The model under review builds one solid part; all positions refer to its coordinate system, in mm. A direction names the side the tool comes from. Round coordinates to 2 decimals unless told otherwise and drop trailing zeros. Order: outer loops, then holes, each group sorted by start corner. A loop starts at its lowest first (then second) coordinate and runs counter-clockwise, first axis right, second up.
```python
from build123d import *

# Parameters (mm, degrees)
SKETCH_1_R           = 22
SKETCH_1_R_2         = 17
EXTRUDE_1_DEPTH      = 9
SKETCH_2_R           = 22
EXTRUDE_2_DEPTH      = 3
SKETCH_3_R           = 1
CUT_EXTRUDE_1_DEPTH  = 3
CUT_EXTRUDE_2_DEPTH  = 25
SKETCH_5_R           = 4
CUT_EXTRUDE_3_DEPTH  = 10
FILLET_1_R           = 10
FILLET_2_R           = 10
SKETCH_7_R           = 25
SKETCH_7_R_2         = 22
EXTRUDE_3_DEPTH      = 30
EXTRUDE_4_DEPTH      = 4
SKETCH_9_R           = 38.67245247
CUT_EXTRUDE_4_DEPTH  = 1
SKETCH_10_R          = 25
SKETCH_10_R_2        = 22
EXTRUDE_5_DEPTH      = 13.5
SKETCH_11_R          = 23
CUT_EXTRUDE_5_DEPTH  = 10.5
CHAMFER_2_SIZE       = 1
SKETCH_12_R          = 23
CUT_EXTRUDE_6_DEPTH  = 18
SKETCH_13_R          = 39.83087954
CUT_EXTRUDE_7_DEPTH  = 2.5
SKETCH_14_R          = 15
CUT_EXTRUDE_8_DEPTH  = 0.5
SKETCH_15_R          = 25
SKETCH_15_R_2        = 23
EXTRUDE_6_DEPTH      = 2
SKETCH_16_R          = 20
CUT_EXTRUDE_9_DEPTH  = 9
SKETCH_17_R          = 20
SKETCH_17_R_2        = 1
SKETCH_17_R_3        = 4
EXTRUDE_7_DEPTH      = 2.5
SKETCH_18_R          = 1.5
CUT_EXTRUDE_10_DEPTH = 21.5
CUT_EXTRUDE_11_DEPTH = 21.5


with BuildPart() as part:
    # 草图1 → 凸台-拉伸1 (new body)
    with BuildSketch(Plane.XY):
        Circle(SKETCH_1_R)
        Circle(SKETCH_1_R_2, mode=Mode.SUBTRACT)
    extrude(amount=EXTRUDE_1_DEPTH)

    # 草图2 → 凸台-拉伸2 (add)
    with BuildSketch(Plane(origin=(0, 0, 0), x_dir=(-1, 0, 0), z_dir=(0, 0, -1))):
        Circle(SKETCH_2_R)
    extrude(amount=EXTRUDE_2_DEPTH)

    # 草图3 → 切除-拉伸1 (cut)
    with BuildSketch(Plane(origin=(0, 0, -3), x_dir=(-1, 0, 0), z_dir=(0, 0, -1))):
        with Locations((0, 10)):
            Circle(SKETCH_3_R)
        with Locations((8.660254038, -5)):
            Circle(SKETCH_3_R)
        with Locations((-8.660254038, -5)):
            Circle(SKETCH_3_R)
    extrude(amount=-CUT_EXTRUDE_1_DEPTH, mode=Mode.SUBTRACT)

    # 草图4 → 切除-拉伸2 (cut)
    with BuildSketch(Plane(origin=(0, 0, -3), x_dir=(-1, 0, 0), z_dir=(0, 0, -1))):
        Polygon((24.787699458, -8.537682263), (5, 2.886751346), (5, 15), (5, 31.006622637), (28.596284234, 19.54376122), align=None)
        Polygon((-6.160254038, -9.330127019), (0, -5.773502692), (19.787699458, -17.197936301), (-4.03507969, -32.43608202), (-23.902747272, -19.573760264), align=None)
        Polygon((-5, 10), (-5, 2.886751346), (-28.902747272, -10.913506226), (-27.638085306, 27.170625695), (-5, 31.006622637), align=None)
    extrude(amount=-CUT_EXTRUDE_2_DEPTH, mode=Mode.SUBTRACT)

    # 草图5 → 切除-拉伸3 (cut)
    with BuildSketch(Plane(origin=(0, 0, -3), x_dir=(-1, 0, 0), z_dir=(0, 0, -1))):
        Circle(SKETCH_5_R)
    extrude(amount=-CUT_EXTRUDE_3_DEPTH, mode=Mode.SUBTRACT)

    # 圆角1
    fillet_1_edges = [part.edges().sort_by_distance(p)[0] for p in [
        (-5, 2.886751346, -1.5),
    ]]
    fillet(fillet_1_edges, radius=FILLET_1_R)

    # 圆角2
    fillet_2_edges = [part.edges().sort_by_distance(p)[0] for p in [
        (5, 2.886751346, -1.5),
        (0, -5.773502692, -1.5),
    ]]
    fillet(fillet_2_edges, radius=FILLET_2_R)

    # 草图7 → 凸台-拉伸3 (add)
    with BuildSketch(Plane(origin=(0, 0, -3), x_dir=(-1, 0, 0), z_dir=(0, 0, -1))):
        Circle(SKETCH_7_R)
        Circle(SKETCH_7_R_2, mode=Mode.SUBTRACT)
    extrude(amount=-EXTRUDE_3_DEPTH)

    # 草图8 → 凸台-拉伸4 (add)
    with BuildSketch(Plane(origin=(0, 0, -3), x_dir=(-1, 0, 0), z_dir=(0, 0, -1))):
        with BuildLine():
            Line((-21.053975315, -6.382015624), (-15.753584421, -3.321833514))
            ThreePointArc((-15.753584421, -3.321833514), (-13.943009001, -8.05), (-10.753584421, -11.982087552))
            Line((-10.753584421, -11.982087552), (-16.053975315, -15.042269662))
            ThreePointArc((-16.053975315, -15.042269662), (-19.052558883, -11), (-21.053975315, -6.382015624))
        make_face()
        with BuildLine():
            Line((16.053975315, -15.042269662), (10.753584421, -11.982087552))
            ThreePointArc((10.753584421, -11.982087552), (13.943009001, -8.05), (15.753584421, -3.321833514))
            Line((15.753584421, -3.321833514), (21.053975315, -6.382015624))
            ThreePointArc((21.053975315, -6.382015624), (19.052558883, -11), (16.053975315, -15.042269662))
        make_face()
        with BuildLine():
            Line((5, 21.424285286), (5, 15.303921066))
            ThreePointArc((5, 15.303921066), (0, 16.1), (-5, 15.303921066))
            Line((-5, 15.303921066), (-5, 21.424285286))
            ThreePointArc((-5, 21.424285286), (0, 22), (5, 21.424285286))
        make_face()
    extrude(amount=EXTRUDE_4_DEPTH)

    # 草图9 → 切除-拉伸4 (cut)
    with BuildSketch(Plane(origin=(0, 0, -7), x_dir=(-1, 0, 0), z_dir=(0, 0, -1))):
        Circle(SKETCH_9_R)
    extrude(amount=-CUT_EXTRUDE_4_DEPTH, mode=Mode.SUBTRACT)

    # 草图10 → 凸台-拉伸5 (add)
    with BuildSketch(Plane(origin=(0, 0, -3), x_dir=(-1, 0, 0), z_dir=(0, 0, -1))):
        Circle(SKETCH_10_R)
        Circle(SKETCH_10_R_2, mode=Mode.SUBTRACT)
    extrude(amount=EXTRUDE_5_DEPTH)

    # 草图11 → 切除-拉伸5 (cut)
    with BuildSketch(Plane(origin=(0, 0, -16.5), x_dir=(-1, 0, 0), z_dir=(0, 0, -1))):
        Circle(SKETCH_11_R)
    extrude(amount=-CUT_EXTRUDE_5_DEPTH, mode=Mode.SUBTRACT)

    # 倒角2
    chamfer_2_edges = [part.edges().sort_by_distance(p)[0] for p in [
        (23, 0, -16.5),
    ]]
    chamfer(chamfer_2_edges, length=CHAMFER_2_SIZE)

    # 草图12 → 切除-拉伸6 (cut)
    with BuildSketch(Plane.XY.offset(27)):
        Circle(SKETCH_12_R)
    extrude(amount=-CUT_EXTRUDE_6_DEPTH, mode=Mode.SUBTRACT)

    # 草图13 → 切除-拉伸7 (cut)
    with BuildSketch(Plane.XY.offset(27)):
        Circle(SKETCH_13_R)
    extrude(amount=-CUT_EXTRUDE_7_DEPTH, mode=Mode.SUBTRACT)

    # 草图14 → 切除-拉伸8 (cut)
    with BuildSketch(Plane(origin=(0, 0, -3), x_dir=(-1, 0, 0), z_dir=(0, 0, -1))):
        Circle(SKETCH_14_R)
    extrude(amount=-CUT_EXTRUDE_8_DEPTH, mode=Mode.SUBTRACT)

    # 草图15 → 凸台-拉伸6 (add)
    with BuildSketch(Plane.XY.offset(24.5)):
        Circle(SKETCH_15_R)
        Circle(SKETCH_15_R_2, mode=Mode.SUBTRACT)
    extrude(amount=EXTRUDE_6_DEPTH)

    # 草图16 → 切除-拉伸9 (cut)
    with BuildSketch(Plane.XY.offset(9)):
        Circle(SKETCH_16_R)
    extrude(amount=-CUT_EXTRUDE_9_DEPTH, mode=Mode.SUBTRACT)

    # 草图17 → 凸台-拉伸7 (add)
    with BuildSketch(Plane.XY):
        Circle(SKETCH_17_R)
        with Locations((8.660254038, -5)):
            Circle(SKETCH_17_R_2, mode=Mode.SUBTRACT)
        with Locations((-8.660254038, -5)):
            Circle(SKETCH_17_R_2, mode=Mode.SUBTRACT)
        with Locations((0, 10)):
            Circle(SKETCH_17_R_2, mode=Mode.SUBTRACT)
        Circle(SKETCH_17_R_3, mode=Mode.SUBTRACT)
    extrude(amount=-EXTRUDE_7_DEPTH)

    # 草图18 → 切除-拉伸10 (cut)
    with BuildSketch(Plane(origin=(0, 0, -2.5), x_dir=(-1, 0, 0), z_dir=(0, 0, -1))):
        with Locations((-6.92603443, -4.003754122)):
            Circle(SKETCH_18_R)
        with Locations((-4.003754122, 6.92603443)):
            Circle(SKETCH_18_R)
        with Locations((6.92603443, 4.003754122)):
            Circle(SKETCH_18_R)
        with Locations((4.003754122, -6.92603443)):
            Circle(SKETCH_18_R)
    extrude(amount=-CUT_EXTRUDE_10_DEPTH, mode=Mode.SUBTRACT)

    # 草图19 → 切除-拉伸11 (cut)
    with BuildSketch(Plane(origin=(0, 0, -2.5), x_dir=(-1, 0, 0), z_dir=(0, 0, -1))):
        with BuildLine():
            Line((-19.986274047, -5.765578009), (-14.740678373, -2.737031935))
            ThreePointArc((-14.740678373, -2.737031935), (-12.983998114, 7.496314806), (-5, 14.134317907))
            Line((-5, 14.134317907), (-5, 20.191410056))
            ThreePointArc((-5, 20.191410056), (-18.014432548, 10.400637481), (-19.986274047, -5.765578009))
        make_face()
        with BuildLine():
            Line((5, 20.191410056), (5, 14.134317907))
            ThreePointArc((5, 14.134317907), (12.983998114, 7.496314806), (14.740678373, -2.737031935))
            Line((14.740678373, -2.737031935), (19.986274047, -5.765578009))
            ThreePointArc((19.986274047, -5.765578009), (18.014432548, 10.400637481), (5, 20.191410056))
        make_face()
        with BuildLine():
            Line((14.986274047, -14.425832047), (9.740678373, -11.397285972))
            ThreePointArc((9.740678373, -11.397285972), (0, -14.992629613), (-9.740678373, -11.397285972))
            Line((-9.740678373, -11.397285972), (-14.986274047, -14.425832047))
            ThreePointArc((-14.986274047, -14.425832047), (0, -20.801274962), (14.986274047, -14.425832047))
        make_face()
    extrude(amount=-CUT_EXTRUDE_11_DEPTH, mode=Mode.SUBTRACT)


solid = part.part
```
(1) Consider section A-A (x = 0). State how many separate pieces and enclosed holes the cut face has, and give its area (3 significant figures).
Data:
separate pieces: 4
enclosed holes: 0
area: 308 mm2
(2) Consider section B-B (y = 0). Write out the cut boundary in (x, z), and give its area (3 significant figures).
Data:
outline: (-25, -16.5) - (-24, -16.5) - (-23, -15.5) - (-23, -6) - (-22, -6) - (-22, 9) - (-23, 9) - (-23, 26.5) - (-25, 26.5) - close; (-14.99, -2.5) - (-4, -2.5) - (-4, 0) - (-14.99, 0) - close; (4, -2.5) - (14.99, -2.5) - (14.99, 0) - (4, 0) - close; (22, -6) - (23, -6) - (23, -15.5) - (24, -16.5) - (25, -16.5) - (25, 26.5) - (23, 26.5) - (23, 9) - (22, 9) - close
area: 256 mm2
(3) Insertion check: pin 1 (5 mm diameter, centred on x = 0, y = 0, fed in from +Z); pin 2 (2 mm diameter, centred on y = -3.5, z = 0, fed in from +X); pin 3 (2 mm diameter, centred on y = 19.5, z = 2, fed in from -X); pin 4 (8 mm diameter, centred on x = 12.5, z = 7.5, fed in from +Y). Each pin has a flat end and moves straight along its axis. Give the tip position at first contact, or say it passes through.
Data:
pin 1: passes through
pin 2: stops at x = 24.87
pin 3: stops at x = -16.82
pin 4: stops at y = 23.51
(4) To check wall thickness, follow probe 1 along Y at (x, z) = (0, -1.8); probe 2 along Y at (x, z) = (0, 26); probe 3 along X at (y, z) = (10, -0.85). State the ranges of each line that lie inside material, in increasing order.
Data:
probe 1: y = -25 to -22, -14.99 to -4, 4 to 9, 11 to 25
probe 2: y = -25 to -23, 23 to 25
probe 3: x = -22.91 to -19.6, -11.17 to -1, 1 to 11.17, 19.6 to 22.91
(5) Draft analysis for pull direction Y (two halves, no side actions). For faces 4 (the cylindrical face through (-17.356, -9.939, 4.563)), 5 (the flat face through (9.4, 22.3, -16.5)), state which applies: pulls with the +Y half, pulls with the -Y half, needs draft (parallel to the pull), parting line crosses it, or undercut.
Data:
face 4: undercut
face 5: needs draft
(6) For faces 1 (the cylindrical face through (-0.15, -14.99, -1.27)), 2 (the flat face through (-12, -12, -6)), 3 (the flat face through (15, -14, 9)), list the 3-axis set-ups (+Z, -Z, +X, -X, +Y, -Y) from which the entire face can be reached by the end or side of a thin tool; tool diameter is ignored.
Data:
face 1: +Z, -Z
face 2: -Z
face 3: +Z
(7) Consider section C-C (z = 16.5). Write out the cut boundary in (x, y), and give its area (3 significant figures).
Data:
outline: circle Ø50 at (0, 0); hole circle Ø46 at (0, 0)
area: 302 mm2
